Build history of the part. All positions in model axes, mm. Face numbers are marked on the shaded views. A direction names the side the tool comes from. Give positions to 0.01 mm unless a question says otherwise; leave off trailing zeros. Order: outer loops, then holes, each group sorted by start corner. A loop starts at its lowest first (then second) coordinate and runs counter-clockwise, first axis right, second up. Notation, with made-up numbers: M 69,10 L 110,10 A21 cw 110,33 Z; hole C -13.5,59 d5. An arc over 180 degrees is marked long. One line per item, written item: value. Start each with the question number.
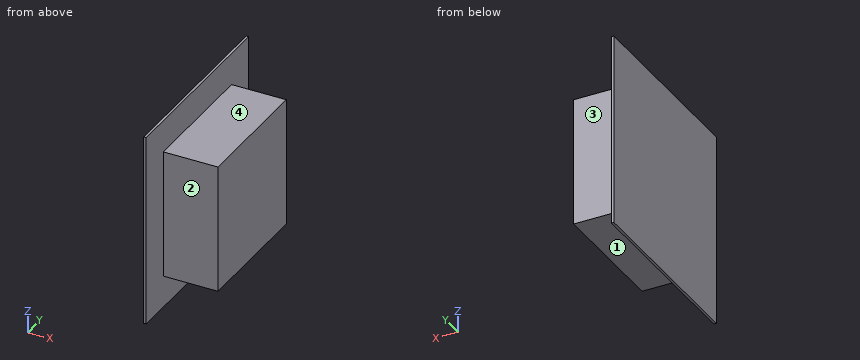
from build123d import *

# Parameters (mm, degrees)
F0_W     = 180
F0_H     = 180
F1_DEPTH = 2.3
F2_W     = 120
F2_H     = 120
F3_DEPTH = 51


with BuildPart() as f1:
    # F0 (on Right) → F1 (new body)
    with BuildSketch(Plane.YZ):
        Rectangle(F0_W, F0_H)
    extrude(amount=F1_DEPTH)

    # F2 (on face) → F3 (join)
    with BuildSketch(Plane.YZ.offset(2.3)):
        Rectangle(F2_W, F2_H)
    extrude(amount=F3_DEPTH)


solid = f1.part
1) Drill centre lines: line 1 (Y direction, x = 5, z = -34); line 2 (X direction, y = -65, z = 66). Where is each one in solid material? Low to high.
2) Tool access for the marked faces 1, 2, 3 and 4: list every direction of +Z, -Z, +X, -X, +Y, -Y with a clear straight run to the whole face (end or side of a thin tool).
3) Drop flat-ended pins along their axis: P1, Ø1, axis at x = 19, y = -11, coming from the +Z side; P2, Ø2, axis at x = 44.5, y = 54.5, coming from the -Z side; P3, Ø1.5, axis at y = -39.5, z = 66.5, coming from the +X side. Give the stop position or say it passes through.
4) Slice it at D-D (z = 73). List the corners of the cut face in (x, y).
5) Slice it at C-C (x = 25.5). List the corners of the cut face in (y, z).
6) Slice it at A-A (y = -35.5). List the corners of the cut face in (x, z).
Results list:
1. line 1: y = -60 to 60
1. line 2: x = 0 to 2.3
2. face 1: -Z, +X, +Y, -Y
2. face 2: +Z, -Z, +X, -Y
2. face 3: +Z, -Z, +X, +Y
2. face 4: +Z, +X, +Y, -Y
3. P1: stops at z = 60
3. P2: stops at z = -60
3. P3: stops at x = 2.3
4. outline: M 0,-90 L 2.3,-90 L 2.3,90 L 0,90 Z
5. outline: M -60,-60 L 60,-60 L 60,60 L -60,60 Z
6. outline: M 0,-90 L 2.3,-90 L 2.3,-60 L 53.3,-60 L 53.3,60 L 2.3,60 L 2.3,90 L 0,90 Z
